```python
from build123d import *

# Parameters (mm, degrees)
BOSS_EXTRUDE1_DEPTH = 6.35


with BuildPart() as part:
    # Sketch1 → Boss-Extrude1 (new body)
    with BuildSketch(Plane(origin=(0, 0, 0), x_dir=(1, 0, 0), z_dir=(0, 1, 0))):
        with BuildLine():
            Line((0, 0), (0, 7.57119509))
            Line((0, 7.57119509), (65.278, 7.57119509))
            ThreePointArc((65.278, 7.57119509), (63.993935294, 7.375852222), (62.826050709, 6.807497929))
            Line((62.826050709, 6.807497929), (43.381923411, -6.606107017))
            ThreePointArc((43.381923411, -6.606107017), (40.638946364, -7.262106405), (38.168659449, -5.901246074))
            Line((38.168659449, -5.901246074), (28.862380436, 5.189545373))
            ThreePointArc((28.862380436, 5.189545373), (27.553926685, 6.193557249), (25.943751107, 6.55052458))
            Line((25.943751107, 6.55052458), (7.147751107, 6.55052458))
            ThreePointArc((7.147751107, 6.55052458), (5.628517155, 6.234523464), (4.361293504, 5.338938332))
            Line((4.361293504, 5.338938332), (0.896741835, 1.623661528))
            ThreePointArc((0.896741835, 1.623661528), (0.348055551, 0.867234544), (0, 0))
        make_face()
    extrude(amount=BOSS_EXTRUDE1_DEPTH)


solid = part.part
```
CAD build for the part. Positions are in the model's coordinates, mm. A direction names the side the tool comes from. Give positions to 0.01 mm unless a question says otherwise; leave off trailing zeros. Order: outer loops, then holes, each group sorted by start corner. A loop starts at its lowest first (then second) coordinate and runs counter-clockwise, first axis right, second up.
(1) Drill centre lines: L1, parallel to X at y = 4.75, z = -3.25; L2, parallel to Z at x = 25, y = 5; L3, parallel to X at y = 2.75, z = -4.5. Where is each one in solid material? Low to high.
(2) Tool access for faces 1 (the cylindrical face through (5.649, 3.131, -6.243)), 2 (the flat face through (53.24, 3.131, -0.195)): list every direction of +Z, -Z, +X, -X, +Y, -Y with a clear straight run to the whole face (end or side of a thin tool).
(3) Saw through at A-A, the plane z = -4.5. Give the cut face in (x, y), then the cut area to 3 significant figures.
(4) Flat gauge pins, fed straight in: pin 1 (3 mm diameter, centred on x = 17, y = 5.5, fed in from +Z); pin 2 (1 mm diameter, centred on x = 47, y = 5.5, fed in from +Z); pin 3 (3 mm diameter, centred on y = 4.5, z = 4, fed in from +X). Where does each tip first touch, or does it go through?
(5) Saw through at D-D, the plane z = 1. Give the cut face in (x, y), then the cut area to 3 significant figures.
(6) Mould opens along X. For faces 3 (the cylindrical face through (64.01, 3.13, -7.38)), 4 (the flat face through (40, 0, -4)), 5 (the cylindrical face through (27.575, 3.131, -6.184)) say: released by +X, released by -X, zero draft, split by the parting line, or undercut.
(7) Saw through at B-B, the plane y = 2. Give the cut face in (x, z).
(8) Saw through at C-C, the plane x = 36. Give the cut face in (y, z), then the cut area to 3 significant figures.
Results found:
1. L1: x = 0 to 2.41, 30.49 to 57.67
1. L2: z = -7.57 to -6.55
1. L3: x = 0 to 3.58, 29.44 to 59.48
2. face 1: +Z, +Y, -Y
2. face 2: +Z, +X, +Y, -Y
3. outline: (0, 0) - (3.58, 0) - (3.58, 6.35) - (0, 6.35) - close; (29.44, 0) - (59.48, 0) - (59.48, 6.35) - (29.44, 6.35) - close
3. area: 213 mm2
4. pin 1: stops at z = -6.55
4. pin 2: stops at z = 4.46
4. pin 3: stops at x = 49.33
5. outline: (34.06, 0) - (51.51, 0) - (51.51, 6.35) - (34.06, 6.35) - close
5. area: 111 mm2
6. face 3: released by +X
6. face 4: zero draft
6. face 5: undercut
7. outline: (0, -7.57) - (65.28, -7.57) arc R4.32 cw to (62.83, -6.81) - (43.38, 6.61) arc R3.91 ccw to (38.17, 5.9) - (28.86, -5.19) arc R3.81 cw to (25.94, -6.55) - (7.15, -6.55) arc R3.81 cw to (4.36, -5.34) - (0.9, -1.62) arc R3.81 cw to (0, 0) - close
8. outline: (0, -7.57) - (6.35, -7.57) - (6.35, 3.32) - (0, 3.32) - close
8. area: 69.1 mm2
